Design review of the part built by this model. Coordinates are the model's own, in mm. Face numbers are marked on the shaded views. A direction names the side the tool comes from. Give positions to 0.01 mm unless a question says otherwise; leave off trailing zeros. Loops run counter-clockwise (first coordinate to the right, second up) from the corner with the lowest first, then second, coordinate; pieces in that order, holes last. Notation, with made-up numbers: (13.5, -37.5) -> (33.5, -37.5) arc R15 cw to (33.5, -10.5) -> close; hole circle Ø1 at (-18.75, -29.5). An arc over 180 degrees is marked (long way). Answer in a Markdown table with one row per item. Add a question column.
(1) For pin 1 (2 mm diameter, centred on x = -12.5, y = -18.5, fed in from +Z); pin 2 (2 mm diameter, centred on x = -13, z = 5.5, fed in from -Y); pin 3 (3.5 mm diameter, centred on x = 66, z = 6.5, fed in from +Y), all flat-tipped, find the tip position at first contact; note any pin that passes through.
(2) Consider section C-C on y = -0.5. Write out the cut boundary in (x, z), then the cut area to 3 significant figures.
(3) For line 1 (Y direction, x = 42.5, z = 11); line 2 (X direction, y = -6, z = 0.5); line 3 (X direction, y = 14, z = 5), list the stretches that pass through material, from the lowest coordinate up.
(4) For the marked faces 5 and 6, list the 3-axis set-ups (+Z, -Z, +X, -X, +Y, -Y) from which the entire face can be reached by the end or side of a thin tool; tool diameter is ignored.
(5) Draft analysis for pull direction X (two halves, no side actions). For the marked faces 1, 2, 3 and 4, state which applies: +X half, -X half, draft (parallel to the pull), parting line (faces both ways), or undercut.
(6) Consider section D-D on x = 1.5. Write out the cut boundary in (y, z).
(7) Consider section B-B on x = -52. Write out the cut boundary in (y, z) (3 decimals), then the cut area to 3 significant figures.
(8) Consider section A-A on x = 43. Write out the cut boundary in (y, z).
from build123d import *

# Parameters (mm, degrees)
F0_R           = 8
F0_R_2         = 10
F0_R_3         = 6
F0_R_4         = 2.455
F1_DEPTH       = 12
F2_R           = 10
F3_DEPTH       = 8
F5_D           = 4.91
F5_DEPTH       = 20
F5_TIP         = 1.4751128197
F6_D           = 4.91
F6_DEPTH       = 21
F6_TIP         = 1.4751128197
F8_D           = 6.6
F8_DEPTH       = 21
F8_CBORE_D     = 11.25
F8_CBORE_DEPTH = 6
F8_TIP         = 1.9828400428


with BuildPart() as f1:
    # F0 (on Top) → F1 (new body)
    with BuildSketch(Plane.XY):
        with BuildLine():
            Line((-73, -25), (73, -25))
            Line((73, -25), (73, -3.9333401471))
            Line((73, -3.9333401471), (58.0210311287, -3.9333401471))
            ThreePointArc((58.0210311287, -3.9333401471), (27.9501482812, -3.0668074952), (58.0121529688, -1.9333401471))
            Line((58.0121529688, -1.9333401471), (73, -1.9333401471))
            Line((73, -1.9333401471), (73, 25))
            Line((73, 25), (-73, 25))
            Line((-73, 25), (-73, -25))
        make_face()
        with Locations((-52, -3)):
            Circle(F0_R, mode=Mode.SUBTRACT)
        with Locations((-22, -3)):
            Circle(F0_R_2, mode=Mode.SUBTRACT)
        with Locations((8, -3)):
            Circle(F0_R, mode=Mode.SUBTRACT)
        with Locations((-63, 10)):
            Circle(F0_R_3, mode=Mode.SUBTRACT)
        with Locations((-38, 10)):
            Circle(F0_R_4, mode=Mode.SUBTRACT)
        with Locations((-6, 10)):
            Circle(F0_R_4, mode=Mode.SUBTRACT)
    extrude(amount=F1_DEPTH)

    # F2 (on face) → F3 (cut)
    with BuildSketch(Plane.XY.offset(12)):
        with BuildLine():
            Line((-6, -25), (-6, -3))
            ThreePointArc((-6, -3), (-22, 13), (-38, -3))
            Line((-38, -3), (-38, -25))
            Line((-38, -25), (-6, -25))
        make_face()
        with Locations((-22, -3)):
            Circle(F2_R, mode=Mode.SUBTRACT)
    extrude(amount=-F3_DEPTH, mode=Mode.SUBTRACT)

    # F5
    with Locations(Plane.XZ.offset(25)):
        with Locations((-52, 6), (8, 6)):
            Hole(F5_D / 2, depth=F5_DEPTH)
            with Locations((0, 0, -(F5_DEPTH + F5_TIP / 2))):  # 118° drill point
                Cone(0, F5_D / 2, F5_TIP, mode=Mode.SUBTRACT)

    # F6
    with Locations(Plane.XZ.offset(25)):
        with Locations((66, 6)):
            Hole(F6_D / 2, depth=F6_DEPTH)
            with Locations((0, 0, -(F6_DEPTH + F6_TIP / 2))):  # 118° drill point
                Cone(0, F6_D / 2, F6_TIP, mode=Mode.SUBTRACT)

    # F8
    with Locations(Plane(origin=(0, 25, 0), x_dir=(-1, 0, 0), z_dir=(0, 1, 0))):
        with Locations((-66, 6)):
            CounterBoreHole(F8_D / 2, F8_CBORE_D / 2, F8_CBORE_DEPTH, depth=F8_DEPTH)
            with Locations((0, 0, -(F8_DEPTH + F8_TIP / 2))):  # 118° drill point
                Cone(0, F8_D / 2, F8_TIP, mode=Mode.SUBTRACT)


solid = f1.part
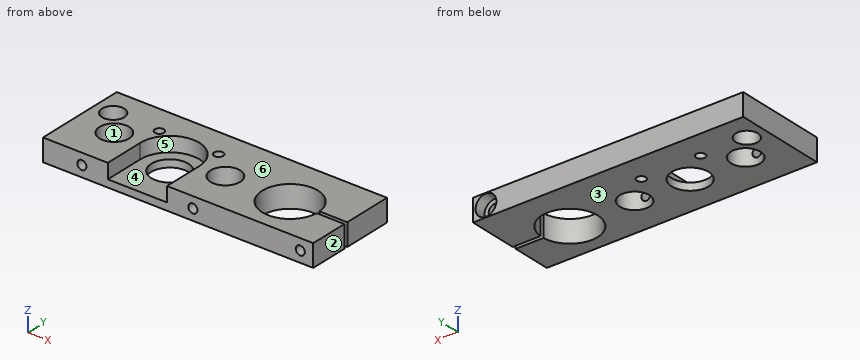
Values follow:
| question | item | result |
|---|---|---|
| 1 | pin 1 | z = 4 |
| 1 | pin 2 | y = 9.49 |
| 1 | pin 3 | y = 3.37 |
| 2 | outline | (-73, 0) -> (-59.6, 0) -> (-59.6, 12) -> (-73, 12) -> close; (-44.4, 0) -> (-31.68, 0) -> (-31.68, 4) -> (-37.8, 4) -> (-37.8, 12) -> (-44.4, 12) -> close; (-12.32, 0) -> (0.4, 0) -> (0.4, 12) -> (-6.2, 12) -> (-6.2, 4) -> (-12.32, 4) -> close; (15.6, 0) -> (28.16, 0) -> (28.16, 12) -> (15.6, 12) -> close; (57.84, 0) -> (73, 0) -> (73, 12) -> (57.84, 12) -> close |
| 2 | area | 701 mm2 |
| 3 | line 1 | -25 to -18.04, 12.04 to 25 |
| 3 | line 2 | -73 to -59.42, -44.58 to -31.54, -12.46 to 0.58, 15.42 to 28.25, 57.75 to 73 |
| 3 | line 3 | -73 to -67.47, -58.53 to 62.86, 69.14 to 73 |
| 4 | face 5 | +Z, -Y |
| 4 | face 6 | +Z, +X, -X, +Y, -Y |
| 5 | face 1 | undercut |
| 5 | face 2 | +X half |
| 5 | face 3 | draft |
| 5 | face 4 | undercut |
| 6 | outline | (-25, 0) -> (-7.66, 0) -> (-7.66, 12) -> (-25, 12) -> close; (1.66, 0) -> (25, 0) -> (25, 12) -> (1.66, 12) -> close |
| 7 | outline | (-25, 0) -> (-11, 0) -> (-11, 3.545) -> (-25, 3.545) -> close; (-25, 8.455) -> (-11, 8.455) -> (-11, 12) -> (-25, 12) -> close; (5, 0) -> (25, 0) -> (25, 12) -> (5, 12) -> close |
| 7 | area | 339 mm2 |
| 8 | outline | (-25, 0) -> (-18.05, 0) -> (-18.05, 12) -> (-25, 12) -> close; (12.05, 0) -> (25, 0) -> (25, 12) -> (12.05, 12) -> close |
